Geometry: final body of the model. Coordinates: model frame, mm. A direction names the side the tool comes from. Coordinates: 2 decimals unless noted, no trailing zeros. Order: outer loops, then holes, each group sorted by start corner. A loop starts at its lowest first (then second) coordinate and runs counter-clockwise, first axis right, second up. Notation, with made-up numbers: M -22,15.25 L 34,15.25 A9 cw 34,19.25 Z; hole C -15,-29 d7. An arc over 180 degrees is marked long. Use CSV: the item, a comma, the result in double quotes. Start each with the question number.
1. Section query B-B on x = 0. Return the cut outline in (y, z).
2. Set-up query: faces 1 (the cylindrical face through (0.88, -12.97, 0.91)), 2 (the flat face through (15, 6, 4)), 3 (the flat face through (23.5, 0, 4)), 4 (the flat face through (-18, 0, 5)). Return all of +Z, -Z, +X, -X, +Y, -Y with unobstructed straight access to the full face (end or side cutting, diameter ignored); none if empty.
3. First-contact query: P1, Ø1, axis at y = -4.5, z = 6.5, coming from the -X side; P2, Ø4, axis at y = 0.5, z = 4.5, coming from the -X side; P3, Ø2, axis at y = 0.5, z = 5.5, coming from the +X side. Flat tips, straight axial feed; report the tip coordinate or a pass-through.
4. Material intervals for line 1 (Y direction, x = -27.3, z = 2.5); line 2 (Y direction, x = -20, z = 3.25); line 3 (Z direction, x = 2, y = -20), sorted ascending.
5. Section query A-A on z = 6.75. Return the cut outline in (x, y).
6. Section query C-C on y = 22.5. Return the cut outline in (x, z).
7. Pull-direction query (Y, two-part tool) for faces 5 (the flat face through (-23, -7.8, 5)), 6 (the cylindrical face through (-8.67, -39.05, 0.89)), 7 (the cylindrical face through (0.678, -17.987, 0.913)), 8 (the flat face through (17, 0, 5.4)); classes: pulls with the +Y half, pulls with the -Y half, needs draft (parallel to the pull), parting line crosses it, or undercut.
from build123d import *

# Parameters (mm, degrees)
SKETCH_R        = 40
PAD_DEPTH       = 1.8
POCKET_DEPTH    = 1.801
SKETCH002_W     = 17.5
SKETCH002_H     = 12
SKETCH002_W_2   = 12.3
SKETCH002_H_2   = 15.6
PAD001_DEPTH    = 3.6
SKETCH003_W     = 4.1
SKETCH003_H     = 12
PAD002_DEPTH    = 3.5
POCKET001_DEPTH = 7.1
SKETCH005_R     = 0.75
POCKET002_DEPTH = 5
SKETCH006_R     = 0.75
POCKET003_DEPTH = 5
SKETCH007_W     = 4.1
SKETCH007_H     = 15.6
PAD003_DEPTH    = 3.5
SKETCH008_R     = 0.75
POCKET004_DEPTH = 8
POCKET005_DEPTH = 1.801


with BuildPart() as part:
    # Sketch → Pad (new body)
    with BuildSketch(Plane.XY):
        Circle(SKETCH_R)
    extrude(amount=PAD_DEPTH)

    # Sketch001 → Pocket (cut, through all)
    with BuildSketch(Plane.XY.offset(1.8)):
        with BuildLine():
            ThreePointArc((-3.886947, -0.944269), (4, 0), (-3.886947, 0.944269))
            ThreePointArc((-3.886947, 0.944269), (-7.65, 0), (-3.886947, -0.944269))
        make_face()
    extrude(amount=-POCKET_DEPTH, mode=Mode.SUBTRACT)

    # Sketch002 → Pad001 (new body)
    with BuildSketch(Plane.XY.offset(1.8)):
        with Locations((14.75, 0)):
            Rectangle(SKETCH002_W, SKETCH002_H)
        with Locations((-24.15, 0)):
            Rectangle(SKETCH002_W_2, SKETCH002_H_2)
    extrude(amount=PAD001_DEPTH)

    # Sketch003 → Pad002 (new body)
    with BuildSketch(Plane.XY.offset(5.4)):
        with Locations((8.05, 0)):
            Rectangle(SKETCH003_W, SKETCH003_H)
    extrude(amount=PAD002_DEPTH)

    # Sketch004 → Pocket001 (cut)
    with BuildSketch(Plane.XY.offset(8.9)):
        with BuildLine():
            ThreePointArc((6, -2.5), (6.5, 0), (6, 2.5))
            Line((6, 2.5), (6, -2.5))
        make_face()
    extrude(amount=-POCKET001_DEPTH, mode=Mode.SUBTRACT)

    # Sketch005 → Pocket002 (cut)
    with BuildSketch(Plane.XY.offset(5.4)):
        with Locations((-27.3, 3.5)):
            Circle(SKETCH005_R)
        with Locations((-27.3, -3.5)):
            Circle(SKETCH005_R)
        with Locations((18.5, 3.5)):
            Circle(SKETCH005_R)
        with Locations((18.5, -3.5)):
            Circle(SKETCH005_R)
    extrude(amount=-POCKET002_DEPTH, mode=Mode.SUBTRACT)

    # Sketch006 → Pocket003 (cut)
    with BuildSketch(Plane.XY.offset(8.9)):
        with Locations((8, 0)):
            Circle(SKETCH006_R)
    extrude(amount=-POCKET003_DEPTH, mode=Mode.SUBTRACT)

    # Sketch007 → Pad003 (new body)
    with BuildSketch(Plane.XY.offset(5.4)):
        with Locations((-20.05, 0)):
            Rectangle(SKETCH007_W, SKETCH007_H)
    extrude(amount=PAD003_DEPTH)

    # Sketch008 → Pocket004 (cut)
    with BuildSketch(Plane.XY.offset(8.9)):
        with Locations((-20, 0)):
            Circle(SKETCH008_R)
    extrude(amount=-POCKET004_DEPTH, mode=Mode.SUBTRACT)

    # Sketch009 → Pocket005 (cut, through all)
    with BuildSketch(Plane.XY.offset(1.8)):
        with BuildLine():
            ThreePointArc((16.970563, 6), (0.974684, 17.973591), (-16.222207, 7.8))
            Line((-16.222207, 7.8), (-10.4, 7.8))
            ThreePointArc((11.532563, 6), (1.063332, 12.95644), (-10.4, 7.8))
            Line((11.532563, 6), (16.970563, 6))
        make_face()
        with BuildLine():
            ThreePointArc((-10.4, -7.8), (1.063332, -12.95644), (11.532563, -6))
            Line((11.532563, -6), (16.970563, -6))
            ThreePointArc((-16.222207, -7.8), (0.974684, -17.973591), (16.970563, -6))
            Line((-16.222207, -7.8), (-10.4, -7.8))
        make_face()
    extrude(amount=-POCKET005_DEPTH, mode=Mode.SUBTRACT)


solid = part.part
Results list:
1,outline,"M -40,0 L -18,0 L -18,1.8 L -40,1.8 Z; M -13,0 L -4,0 L -4,1.8 L -13,1.8 Z; M 4,0 L 13,0 L 13,1.8 L 4,1.8 Z; M 18,0 L 40,0 L 40,1.8 L 18,1.8 Z"
2,face 1,"+Z, -Z"
2,face 2,"+Z"
2,face 3,"+Z, +X, +Y, -Y"
2,face 4,"+Z, +Y, -Y"
3,P1,"stops at x = -22.1"
3,P2,"stops at x = -30.3"
3,P3,"stops at x = 23.5"
4,line 1,"y = -7.8 to -4.25, -2.75 to 2.75, 4.25 to 7.8"
4,line 2,"y = -7.8 to -0.75, 0.75 to 7.8"
4,line 3,"z = 0 to 1.8"
5,outline,"M -22.1,-7.8 L -18,-7.8 L -18,7.8 L -22.1,7.8 Z; M 6,-6 L 10.1,-6 L 10.1,6 L 6,6 L 6,2.5 A6.5 cw 6,-2.5 Z; hole C -20,0 d1.5; hole C 8,0 d1.5"
6,outline,"M -33.07,0 L 33.07,0 L 33.07,1.8 L -33.07,1.8 Z"
7,face 5,"pulls with the -Y half"
7,face 6,"parting line crosses it"
7,face 7,"undercut"
7,face 8,"needs draft"
